For this review, take the finished solid that the model builds, in its own axes (mm). A direction names the side the tool comes from. Coordinates: 2 decimals unless noted, no trailing zeros. Loops run counter-clockwise (first coordinate to the right, second up) from the corner with the lowest first, then second, coordinate; pieces in that order, holes last. Notation, with made-up numbers: (85, 19.25) - (123, 19.25) arc R17 ccw to (123, 48.25) - close; hole circle Ø4 at (39, -13). An arc over 180 degrees is marked (long way). Answer as a JSON object with one key per item and string values. Group by question number.
Item 1: Tool access review of faces 1 (the flat face through (-26, -6, 6.35)), 2 (the flat face through (-25, 0, 59)): name each direction out of +Z, -Z, +X, -X, +Y, -Y from which nothing blocks a thin tool from reaching the whole face with its end or side.
Item 2: We need section D-D (x = -8). Give the boundary of the cut face in (y, z).
Item 3: Mouldability with a two-part tool opening along X and no side actions: class faces 3 (the flat face through (-6.35, -6, 38)), 4 (the flat face through (-26, -25.4, 39)), 5 (the flat face through (-44.45, -6, 38)), 6 (the flat face through (-50.8, -13, 38)) as released by +X, released by -X, zero draft, split by the parting line, or undercut.
Item 4: We need section B-B (z = 68). Give the boundary of the cut face in (x, y), then the cut area to 3 significant figures.
Item 5: We need section A-A (y = -4.5). Give the boundary of the cut face in (x, z), then the cut area to 3 significant figures.
Item 6: We need section C-C (x = -25.4). Give the boundary of the cut face in (y, z), then the cut area to 3 significant figures.
Item 7: To check wall thickness, follow line 1 (X direction, y = -1.25, z = 21.5); line 2 (X direction, y = -5, z = 56); line 3 (Z direction, x = -10.5, y = -6). State the ranges of each line that lie inside material, in increasing order.
from build123d import *

# Parameters (mm, degrees)
F0_W     = 50.8
F0_H     = 76.2
F1_DEPTH = 25.4
F2_W     = 38.1
F2_H     = 63.5
F3_DEPTH = 12.7
F4_R     = 6.35
F5_DEPTH = 25.4


with BuildPart() as f1:
    # F0 (on Front) → F1 (new body)
    with BuildSketch(Plane.XZ):
        with Locations((-25.4, 38.1)):
            Rectangle(F0_W, F0_H)
    extrude(amount=F1_DEPTH)

    # F2 (on Front) → F3 (cut)
    with BuildSketch(Plane.XZ):
        with Locations((-25.4, 38.1)):
            Rectangle(F2_W, F2_H)
    extrude(amount=F3_DEPTH, mode=Mode.SUBTRACT)

    # F4 (on Front) → F5 (join)
    with BuildSketch(Plane.XZ):
        with Locations((-25.4, 58.964718)):
            Circle(F4_R)
    extrude(amount=F5_DEPTH)


solid = f1.part
Check sheet entries:
{
 "1": {"face 1": "+Y", "face 2": "+Z, -Z, +X, -X, +Y"},
 "2": {"outline": "(-25.4, 0) - (0, 0) - (0, 6.35) - (-12.7, 6.35) - (-12.7, 69.85) - (0, 69.85) - (0, 76.2) - (-25.4, 76.2) - close"},
 "3": {"face 3": "undercut", "face 4": "zero draft", "face 5": "undercut", "face 6": "released by -X"},
 "4": {"outline": "(-50.8, -25.4) - (0, -25.4) - (0, 0) - (-6.35, 0) - (-6.35, -12.7) - (-44.45, -12.7) - (-44.45, 0) - (-50.8, 0) - close", "area": "806 mm2"},
 "5": {"outline": "(-50.8, 0) - (0, 0) - (0, 76.2) - (-50.8, 76.2) - close; circle Ø12.7 at (-25.4, 58.96); hole (-44.45, 6.35) - (-6.35, 6.35) - (-6.35, 69.85) - (-44.45, 69.85) - close", "area": "1,580 mm2"},
 "6": {"outline": "(-25.4, 0) - (0, 0) - (0, 6.35) - (-12.7, 6.35) - (-12.7, 52.61) - (0, 52.61) - (0, 65.31) - (-12.7, 65.31) - (-12.7, 69.85) - (0, 69.85) - (0, 76.2) - (-25.4, 76.2) - close", "area": "1,290 mm2"},
 "7": {"line 1": "x = -50.8 to -44.45, -6.35 to 0", "line 2": "x = -50.8 to -44.45, -31.02 to -19.78, -6.35 to 0", "line 3": "z = 0 to 6.35, 69.85 to 76.2"}
}
